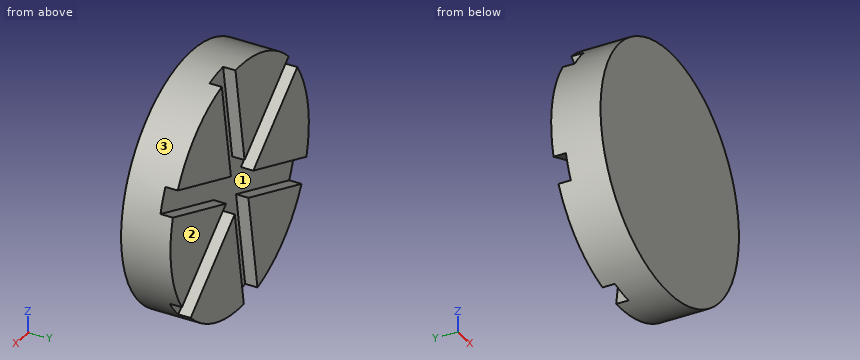
```python
from build123d import *

# Parameters (mm, degrees)
SKETCH1_R           = 127
BOSS_EXTRUDE1_DEPTH = 50.8
CUT_EXTRUDE1_DEPTH  = 12.7


with BuildPart() as part:
    # Sketch1 → Boss-Extrude1 (new body)
    with BuildSketch(Plane(origin=(0, 0, 0), x_dir=(1, 0, 0), z_dir=(0, 1, 0))):
        with Locations(Location((0, 0, 0), (0, 0, 270))):
            Circle(SKETCH1_R)
    extrude(amount=BOSS_EXTRUDE1_DEPTH)

    # Sketch2 → Cut-Extrude1 (cut)
    with BuildSketch(Plane(origin=(0, 50.8, 0), x_dir=(1, 0, 0), z_dir=(0, 1, 0))):
        Polygon((-90.39681042, -90.103865988), (-106.44912427, -70.419272519), (-25.073514933, -4.05941485), (-123.230642135, 33.23400125), (-114.209441053, 56.978009569), (-16.052313851, 19.684593469), (-32.833831715, 123.337867238), (-7.760316782, 127.397282088), (9.021201082, 23.744008319), (90.39681042, 90.103865988), (106.44912427, 70.419272519), (25.073514933, 4.05941485), (123.230642135, -33.23400125), (114.209441053, -56.978009569), (16.052313851, -19.684593469), (32.833831715, -123.337867238), (7.760316782, -127.397282088), (-9.021201082, -23.744008319), align=None)
    extrude(amount=-CUT_EXTRUDE1_DEPTH, mode=Mode.SUBTRACT)


solid = part.part
```
CAD build for the part. Positions are in the model's coordinates, mm. Face numbers are marked on the shaded views. Round coordinates to 2 decimals unless told otherwise and drop trailing zeros. Order: outer loops, then holes, each group sorted by start corner. A loop starts at its lowest first (then second) coordinate and runs counter-clockwise, first axis right, second up. Notation, with made-up numbers: (89, 17) - (103, 17) arc R30 ccw to (103, 54) - close; hole circle Ø10 at (71.25, -3). An arc over 180 degrees is marked (long way). Use CSV: the item, a comma, the result in double quotes. Start each with the question number.
1) Two-plate mould, pull along Z, no slides. Class the marked faces 1, 2 and 3: pulls with the +Z half, pulls with the -Z half, needs draft (parallel to the pull), parting line crosses it, or undercut.
2) Saw through at B-B (z = -52). List the corners of the cut face in (x, y), and give its area (3 significant figures).
3) Saw through at A-A (y = 43.5). List the corners of the cut face in (x, z), and give its area (3 significant figures).
4) Wall check: L1, parallel to Z at x = 57, y = 48.5; L2, parallel to Z at x = -105, y = 41.5; L3, parallel to X at y = 44.5, z = 109.5. Give the ranges that are in metal, low to high. Write a range as [from, to].
5) Saw through at C-C (x = 0). List the corners of the cut face in (y, z), and give its area (3 significant figures).
6) Pin check, flat tips, straight feed: pin 1 Ø3 at (y, z) = (35.5, 32) entering from -X; pin 2 Ø3 at (y, z) = (18, 6.5) entering from +X; pin 3 Ø6 at (x, y) = (-35.5, 16) entering from -Z. Stop position of each tip, or through.
7) Saw through at D-D (y = 27). List the corners of the cut face in (x, z), and give its area (3 significant figures).
Values follow:
1,face 1,"undercut"
1,face 2,"needs draft"
1,face 3,"parting line crosses it"
2,outline,"(-115.87, 0) - (115.87, 0) - (115.87, 50.8) - (83.86, 50.8) - (83.86, 38.1) - (43.67, 38.1) - (43.67, 50.8) - (4.45, 50.8) - (4.45, 38.1) - (-21.28, 38.1) - (-21.28, 50.8) - (-101.11, 50.8) - (-101.11, 38.1) - (-115.87, 38.1) - close"
2,area,"10,700 mm2"
3,outline,"(-122.64, -33.01) - (-25.07, 4.06) - (-105.96, 70.02) arc R127 ccw to start; (-113.61, -56.75) arc R127 ccw to (-32.73, -122.71) - (-16.05, -19.68) - close; (-89.9, 89.7) - (-9.02, 23.74) - (7.66, 126.77) arc R127 ccw to start; (-7.66, -126.77) arc R127 ccw to (89.9, -89.7) - (9.02, -23.74) - close; (16.05, 19.68) - (113.61, 56.75) arc R127 ccw to (32.73, 122.71) - close; (25.07, -4.06) - (105.96, -70.02) arc R127 ccw to (122.64, 33.01) - close"
3,area,"33,000 mm2"
4,L1,"z = [-113.49, -62.87], [-30.09, 8.07], [35.24, 113.49]"
4,L2,"z = [-71.44, -53.48], [-26.31, 69.24]"
4,L3,"x = [-64.33, 4.86], [30.59, 64.33]"
5,outline,"(0, -127) - (50.8, -127) - (50.8, -79.46) - (38.1, -79.46) - (38.1, 79.46) - (50.8, 79.46) - (50.8, 127) - (0, 127) - close"
5,area,"10,900 mm2"
6,pin 1,"stops at x = -123.28"
6,pin 2,"stops at x = 126.9"
6,pin 3,"stops at z = -122.77"
7,outline,"circle Ø254 at (0, 0)"
7,area,"50,700 mm2"
